Here's the drawing with two shaded views (mm, measured from the low corner). I have some questions. Give positions to 0.01 mm unless a question says otherwise; leave off trailing zeros. Loops run counter-clockwise (first coordinate to the right, second up) from the corner with the lowest first, then second, coordinate; pieces in that order, holes last. Notation, with made-up numbers: M 44.5,-29 L 74.5,-29 A11 cw 74.5,-10 Z; hole C 13,16.25 d3. An arc over 180 degrees is marked long. Put each result on its own line as item: value. Start each with the question number.
1) Imagine slicing it at B-B (x = 65.5). Write out the boundary of the cut face in (y, z).
2) Please list where these lines run through material, in increasing order: line 1 along X through (y, z) = (12.5, 1.45); line 2 along Y through (x, z) = (65.5, 2.55); line 3 along X through (y, z) = (14, 4.2). Write a range as from..to.
3) Imagine slicing it at A-A (y = 12.5). Write out the boundary of the cut face in (x, z), then the cut area to 3 significant figures.
4) For P1, Ø2, axis at x = 14.5, y = 12.5, coming from the -Z side, with a flat end and sliding along its axis, tell me the tip position at first contact or that it passes through.
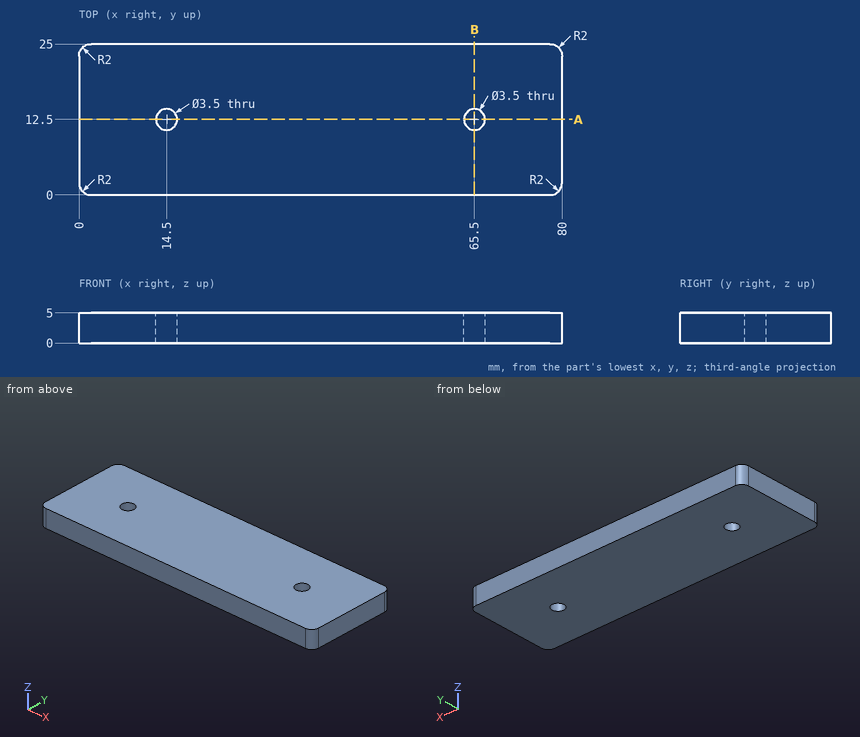
Recorded:
1. outline: M 0,0 L 10.75,0 L 10.75,5 L 0,5 Z; M 14.25,0 L 25,0 L 25,5 L 14.25,5 Z
2. line 1: 0..12.75, 16.25..63.75, 67.25..80
2. line 2: 0..10.75, 14.25..25
2. line 3: 0..13.6, 15.4..64.6, 66.4..80
3. outline: M 0,0 L 12.75,0 L 12.75,5 L 0,5 Z; M 16.25,0 L 63.75,0 L 63.75,5 L 16.25,5 Z; M 67.25,0 L 80,0 L 80,5 L 67.25,5 Z
3. area: 365 mm²
4. P1: through
